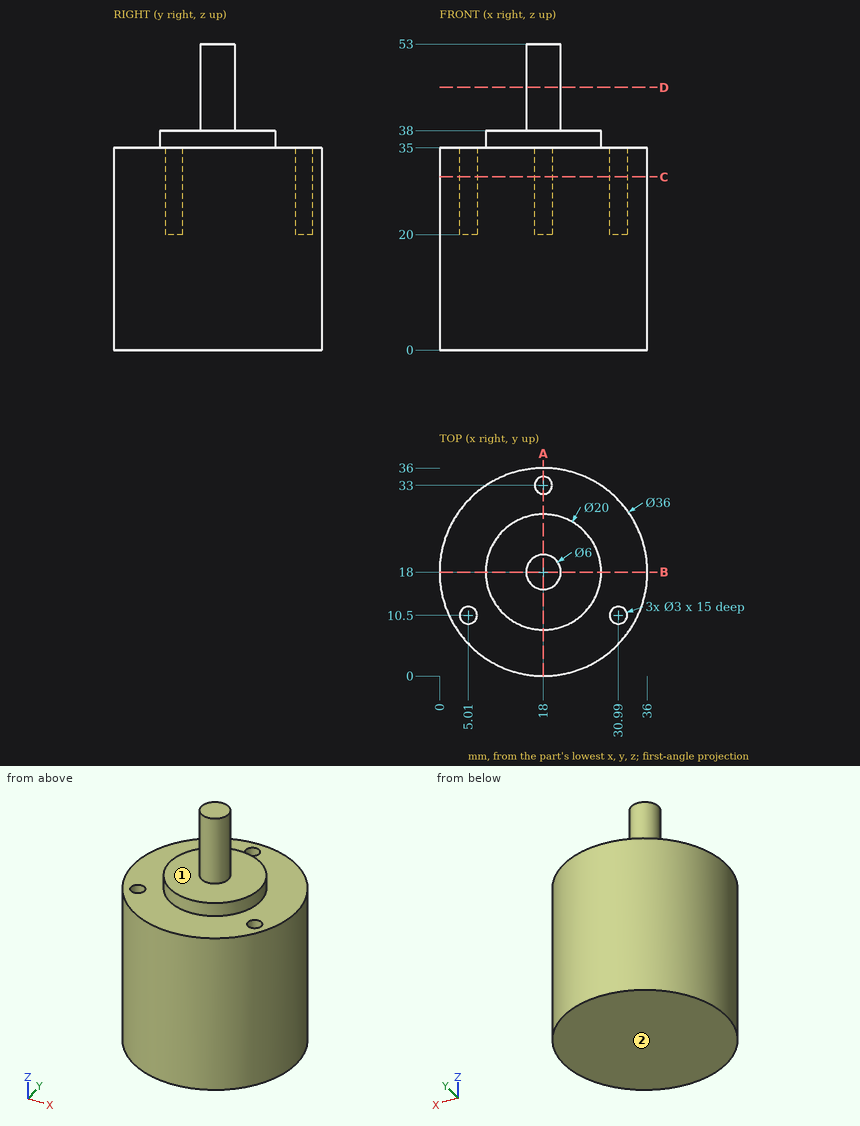
The figure shows three views and two pictorial views of one solid part (mm, origin at its lowest corner). Answer the questions. A direction names the side the tool comes from. Round coordinates to 2 decimals unless told otherwise and drop trailing zeros. Order: outer loops, then holes, each group sorted by start corner. A loop starts at its lowest first (then second) coordinate and runs counter-clockwise, first axis right, second up. Notation, with made-up numbers: (74.25, -18.5) -> (114.25, -18.5) arc R22 ccw to (114.25, 2.5) -> close; hole circle Ø6 at (30.5, 62.25). An arc over 180 degrees is marked (long way). Put each result on its own line as item: value.
Q1. Each of these flat-tipped pins is pushed along its axis until it touches: P1, Ø6, axis at y = 18.5, z = 38.5, coming from the +X side; P2, Ø10, axis at x = 10, y = 29, coming from the +Z side; P3, Ø2.5, axis at x = 18, y = 32.5, coming from the +Z side. Where does it stop, or does it pass through?
Results list:
P1: x = 28
P2: z = 38
P3: z = 35
Q2. Section B-B, the plane y = 18 is taken. Write down the section's boundary in (x, z).
Results list:
outline: (0, 0) -> (36, 0) -> (36, 35) -> (28, 35) -> (28, 38) -> (21, 38) -> (21, 53) -> (15, 53) -> (15, 38) -> (8, 38) -> (8, 35) -> (0, 35) -> close
Q3. Section C-C, the plane z = 30 is taken. Write down the section's boundary in (x, y), and give its area (3 significant figures).
Results list:
outline: circle Ø36 at (18, 18); hole circle Ø3 at (5.01, 10.5); hole circle Ø3 at (18, 33); hole circle Ø3 at (30.99, 10.5)
area: 997 mm^2
Q4. Consider line 1 along Y through (x, z) = (18, 24.5); line 2 along X through (y, z) = (10, 24) (1 decimal); line 3 along Z through (x, y) = (18.5, 15). Determine where each line is inside the solid, lowest interval first.
Results list:
line 1: 0 to 31.5, 34.5 to 36
line 2: 1.9 to 3.6, 6.4 to 29.6, 32.4 to 34.1
line 3: 0 to 38
Q5. Section D-D, the plane z = 45.5 is taken. Write down the section's boundary in (x, y), and give its area (3 significant figures).
Results list:
outline: circle Ø6 at (18, 18)
area: 28.3 mm^2
Q6. Which of the six approach directions +Z, -Z, +X, -X, +Y, -Y give full straight-line access (tool end or side, diameter ignored) to the marked faces 1 and 2?
Results list:
face 1: +Z
face 2: -Z, +X, -X, +Y, -Y
Q7. Section A-A, the plane x = 18 is taken. Write down the section's boundary in (y, z).
Results list:
outline: (0, 0) -> (36, 0) -> (36, 35) -> (34.5, 35) -> (34.5, 20) -> (31.5, 20) -> (31.5, 35) -> (28, 35) -> (28, 38) -> (21, 38) -> (21, 53) -> (15, 53) -> (15, 38) -> (8, 38) -> (8, 35) -> (0, 35) -> close
